The listing builds one solid part. Answer for the finished solid, in the listing's coordinates (mm). Face numbers are marked on the shaded views. Give positions to 0.01 mm unless a question says otherwise; leave off trailing zeros. Loops run counter-clockwise (first coordinate to the right, second up) from the corner with the lowest first, then second, coordinate; pieces in that order, holes last. Notation, with made-up numbers: M -19.5,-37 L 36.5,-37 A37 ccw 36.5,-1 Z; hole C 13,4 d10. An arc over 180 degrees is marked long. Return JSON: item names as keys, results as strings.
from build123d import *

# Parameters (mm, degrees)
SKETCH1_W            = 80
SKETCH1_H            = 30
CHASSIS_DEPTH        = 2
SKETCH2_W            = 3
SKETCH2_H            = 30
TALLVALVEWALL_DEPTH  = 50
SKETCH3_W            = 3
SKETCH3_H            = 30
SHORTVALVEWALL_DEPTH = 30
SKETCH4_R            = 1.5
SKETCH4_R_2          = 3.25
TALLVALVECUT_DEPTH   = 4
SHORTVALVECUT_REACH  = 82
SKETCH6_R            = 3.25
SKETCH6_R_2          = 1.5
TALLVALVELIP_DEPTH   = 3
LIPROUNDING_R        = 3


with BuildPart() as part:
    # Sketch1 → Chassis (new body)
    with BuildSketch(Plane(origin=(0, 0, 0), x_dir=(1, 0, 0), z_dir=(0, 1, 0))):
        Rectangle(SKETCH1_W, SKETCH1_H)
    extrude(amount=CHASSIS_DEPTH)

    # Sketch2 → TallValveWall (add)
    with BuildSketch(Plane(origin=(0, 2, 0), x_dir=(1, 0, 0), z_dir=(0, 1, 0))):
        with Locations((-38.5, 0)):
            Rectangle(SKETCH2_W, SKETCH2_H)
    extrude(amount=TALLVALVEWALL_DEPTH)

    # Sketch3 → ShortValveWall (add)
    with BuildSketch(Plane(origin=(0, 2, 0), x_dir=(1, 0, 0), z_dir=(0, 1, 0))):
        with Locations((38.5, 0)):
            Rectangle(SKETCH3_W, SKETCH3_H)
    extrude(amount=SHORTVALVEWALL_DEPTH)

    # Sketch4 → TallValveCut (cut, through all)
    with BuildSketch(Plane(origin=(-37, 0, 0), x_dir=(0, 0, -1), z_dir=(1, 0, 0))):
        with Locations((-5, 48)):
            Circle(SKETCH4_R)
        with Locations((5, 48)):
            Circle(SKETCH4_R)
        with Locations((5, 38)):
            Circle(SKETCH4_R)
        with Locations((-5, 38)):
            Circle(SKETCH4_R)
        with Locations((0, 43)):
            Circle(SKETCH4_R_2)
    extrude(amount=-TALLVALVECUT_DEPTH, mode=Mode.SUBTRACT)

    # Sketch6 → ShortValveCut (cut, up to next)
    with BuildSketch(Plane(origin=(40, 0, 0), x_dir=(0, 0, -1), z_dir=(1, 0, 0)), mode=Mode.PRIVATE) as shortvalvecut_sk1:
        with Locations((0, 17)):
            Circle(SKETCH6_R)
    shortvalvecut_tool1 = extrude(shortvalvecut_sk1.sketch, amount=-SHORTVALVECUT_REACH, mode=Mode.PRIVATE) & part.part
    add(shortvalvecut_tool1.solids().sort_by_distance((40, 17, 0))[0], mode=Mode.SUBTRACT)
    # Sketch6 → ShortValveCut (cut, up to next)
    with BuildSketch(Plane(origin=(40, 0, 0), x_dir=(0, 0, -1), z_dir=(1, 0, 0)), mode=Mode.PRIVATE) as shortvalvecut_sk2:
        with Locations((0, 24)):
            Circle(SKETCH6_R_2)
    shortvalvecut_tool2 = extrude(shortvalvecut_sk2.sketch, amount=-SHORTVALVECUT_REACH, mode=Mode.PRIVATE) & part.part
    add(shortvalvecut_tool2.solids().sort_by_distance((40, 24, 0))[0], mode=Mode.SUBTRACT)
    # Sketch6 → ShortValveCut (cut, up to next)
    with BuildSketch(Plane(origin=(40, 0, 0), x_dir=(0, 0, -1), z_dir=(1, 0, 0)), mode=Mode.PRIVATE) as shortvalvecut_sk3:
        with Locations((6.657395614, 19.163118961)):
            Circle(SKETCH6_R_2)
    shortvalvecut_tool3 = extrude(shortvalvecut_sk3.sketch, amount=-SHORTVALVECUT_REACH, mode=Mode.PRIVATE) & part.part
    add(shortvalvecut_tool3.solids().sort_by_distance((40, 19.163119, -6.657396))[0], mode=Mode.SUBTRACT)
    # Sketch6 → ShortValveCut (cut, up to next)
    with BuildSketch(Plane(origin=(40, 0, 0), x_dir=(0, 0, -1), z_dir=(1, 0, 0)), mode=Mode.PRIVATE) as shortvalvecut_sk4:
        with Locations((4.114496766, 11.336881039)):
            Circle(SKETCH6_R_2)
    shortvalvecut_tool4 = extrude(shortvalvecut_sk4.sketch, amount=-SHORTVALVECUT_REACH, mode=Mode.PRIVATE) & part.part
    add(shortvalvecut_tool4.solids().sort_by_distance((40, 11.336881, -4.114497))[0], mode=Mode.SUBTRACT)
    # Sketch6 → ShortValveCut (cut, up to next)
    with BuildSketch(Plane(origin=(40, 0, 0), x_dir=(0, 0, -1), z_dir=(1, 0, 0)), mode=Mode.PRIVATE) as shortvalvecut_sk5:
        with Locations((-4.114496766, 11.336881039)):
            Circle(SKETCH6_R_2)
    shortvalvecut_tool5 = extrude(shortvalvecut_sk5.sketch, amount=-SHORTVALVECUT_REACH, mode=Mode.PRIVATE) & part.part
    add(shortvalvecut_tool5.solids().sort_by_distance((40, 11.336881, 4.114497))[0], mode=Mode.SUBTRACT)
    # Sketch6 → ShortValveCut (cut, up to next)
    with BuildSketch(Plane(origin=(40, 0, 0), x_dir=(0, 0, -1), z_dir=(1, 0, 0)), mode=Mode.PRIVATE) as shortvalvecut_sk6:
        with Locations((-6.657395614, 19.163118961)):
            Circle(SKETCH6_R_2)
    shortvalvecut_tool6 = extrude(shortvalvecut_sk6.sketch, amount=-SHORTVALVECUT_REACH, mode=Mode.PRIVATE) & part.part
    add(shortvalvecut_tool6.solids().sort_by_distance((40, 19.163119, 6.657396))[0], mode=Mode.SUBTRACT)

    # Sketch7 → TallValveLip (add)
    with BuildSketch(Plane(origin=(-37, 0, 0), x_dir=(0, 0, -1), z_dir=(1, 0, 0))):
        Polygon((-13, 52), (-10, 52), (-10, 33), (10, 33), (10, 52), (13, 52), (13, 30), (-13, 30), align=None)
    extrude(amount=TALLVALVELIP_DEPTH)

    # LipRounding
    liprounding_edges = [part.edges().sort_by_distance(p)[0] for p in [
        (-35.5, 30, 13),
        (-35.5, 30, -13),
        (-35.5, 33, -10),
        (-35.5, 33, 10),
    ]]
    fillet(liprounding_edges, radius=LIPROUNDING_R)


solid = part.part
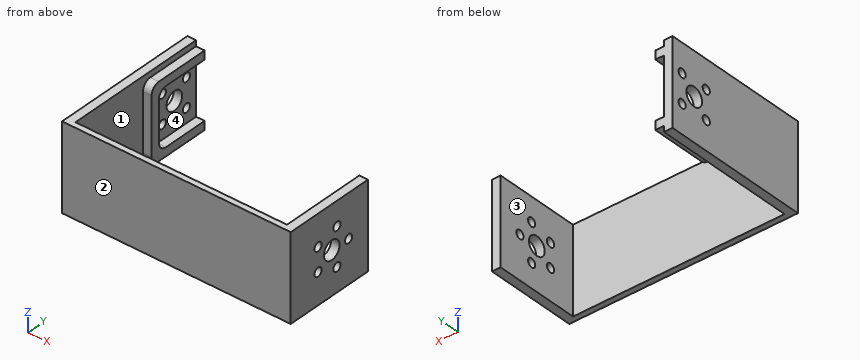
(1) The part is cut by section B-B (y = 24). Determine the outline of the cut face in (x, z).
Values follow:
{"outline": "M -40,-15 L -37,-15 L -37,15 L -40,15 Z; M 37,-15 L 40,-15 L 40,-1.5 L 37,-1.5 Z; M 37,1.5 L 40,1.5 L 40,15 L 37,15 Z"}
(2) Straight lines are drawn through the part: line 1 along Y through (x, z) = (-38.2, 5); line 2 along X through (y, z) = (11.5, 13); line 3 along Y through (x, z) = (-37.8, 0). For each, find the intervals that lie inside material, in ascending order.
Values follow:
{"line 1": "0 to 36.5, 39.5 to 46.5, 49.5 to 52", "line 2": "-40 to -37, 37 to 40", "line 3": "0 to 39.75, 46.25 to 52"}
(3) The part is cut by section A-A (z = 0). Determine the outline of the cut face in (x, y), and give its area (3 significant figures).
Values follow:
{"outline": "M -40,0 L 40,0 L 40,13.75 L 37,13.75 L 37,2 L -37,2 L -37,30 L -34,30 L -34,33 L -37,33 L -37,39.75 L -40,39.75 Z; M -40,46.25 L -37,46.25 L -37,52 L -40,52 Z; M 37,20.25 L 40,20.25 L 40,22.5 L 37,22.5 Z; M 37,25.5 L 40,25.5 L 40,32 L 37,32 Z", "area": "361 mm²"}
(4) Determine the mould class of the marked faces 1, 2, 3 and 4 for opening direction X: released by +X, released by -X, zero draft, split by the parting line, or undercut.
Values follow:
{"face 1": "undercut", "face 2": "zero draft", "face 3": "undercut", "face 4": "released by +X"}
(5) The part is cut by section D-D (x = 33). Determine the outline of the cut face in (y, z).
Values follow:
{"outline": "M 0,-15 L 2,-15 L 2,15 L 0,15 Z"}
(6) Given pin 1 (1.5 mm diameter, centred on x = -36, y = 41.5, fed in from +Z); pin 2 (6 mm diameter, centred on x = -30.5, z = 9.5, fed in from -Y); pin 3 (15 mm diameter, centred on y = 40, z = 1.5, fed in from +X); pin 4 (5 mm diameter, centred on y = 17, z = 0, fed in from +X), each flat-ended and moving along its own axis, determine where each tip first touches the part or whether it passes through.
Values follow:
{"pin 1": "z = 13", "pin 2": "y = 0", "pin 3": "x = -34", "pin 4": "x = -37"}
(7) The part is cut by section C-C (y = 38). Determine the outline of the cut face in (x, z), and give its area (3 significant figures).
Values follow:
{"outline": "M -40,-15 L -37,-15 L -37,-13 L -34,-13 L -34,-10 L -37,-10 L -37,-6.5 L -40,-6.5 Z; M -40,-3.5 L -37,-3.5 L -37,3.5 L -40,3.5 Z; M -40,6.5 L -37,6.5 L -37,10 L -34,10 L -34,13 L -37,13 L -37,15 L -40,15 Z", "area": "90.0 mm²"}
